```python
from build123d import *

# Parameters (mm, degrees)
F0_R           = 63.5
F1_DEPTH       = 12.7
F3_DEPTH       = 25.4
F4_D           = 6.35
F4_CBORE_D     = 10.3124
F4_CBORE_DEPTH = 6.35


# Not quite as in the source:
# - a feature names something its author has since deleted; it is built from what else it names


with BuildPart() as f1:
    # F0 (on Front) → F1 (new body)
    with BuildSketch(Plane.XZ):
        Circle(F0_R)
    extrude(amount=F1_DEPTH)

    # F2 (on face) → F3 (cut)
    with BuildSketch(Plane.XZ.offset(12.7)):
        with BuildLine():
            Line((-10.3124, 62.6570379625), (-6.35, 50.8))
            Line((-6.35, 50.8), (-6.35, -25.4))
            ThreePointArc((-6.35, -25.4), (0, -31.75), (6.35, -25.4))
            Line((6.35, -25.4), (6.35, 50.8))
            Line((6.35, 50.8), (10.3124, 62.6570379625))
            ThreePointArc((10.3124, 62.6570379625), (0, 63.5), (-10.3124, 62.6570379625))
        make_face()
    extrude(amount=-F3_DEPTH, mode=Mode.SUBTRACT)

    # F4 (through all)
    with Locations(Plane(origin=(0, 0, 0), x_dir=(1, 0, 0), z_dir=(0, 1, 0))):
        with Locations((44.45, -29.36875), (-44.45, -29.36875), (44.45, 29.36875), (-44.45, 29.36875)):
            CounterBoreHole(F4_D / 2, F4_CBORE_D / 2, F4_CBORE_DEPTH)


solid = f1.part
```
Work out the finished part from the listing and answer in its coordinate system (mm). A direction names the side the tool comes from. Round coordinates to 2 decimals unless told otherwise and drop trailing zeros. Order: outer loops, then holes, each group sorted by start corner. A loop starts at its lowest first (then second) coordinate and runs counter-clockwise, first axis right, second up.
Q1. A cutting plane is placed at A-A, the plane z = 0. Determine the outline of the cut face in (x, y), then the cut area to 3 significant figures.
Solution:
outline: (-63.5, -12.7) - (-6.35, -12.7) - (-6.35, 0) - (-63.5, 0) - close; (6.35, -12.7) - (63.5, -12.7) - (63.5, 0) - (6.35, 0) - close
area: 1,450 mm2
Q2. A tool of negligible diameter and unlimited length cuts with its end or side. For faces 5 (the cylindrical face through (-39.69, -3.13, -27.39)), 6 (the cylindrical face through (-41.28, -9.57, 29.23)), 7 (the flat face through (8.303, -6.439, 56.646)), from which of +Z, -Z, +X, -X, +Y, -Y can it reach the whole face along a straight path? Write none if from no direction.
Solution:
face 5: +Y
face 6: +Y, -Y
face 7: +Z, +Y, -Y
Q3. Find the intervals of material crossed by line 1 along Z through (x, y) = (-44.45, -9.25); line 2 along Z through (x, y) = (-44.45, -2.5); line 3 along X through (y, z) = (-6, 28), in increasing order.
Solution:
line 1: z = -45.35 to -32.54, -26.19 to 26.19, 32.54 to 45.35
line 2: z = -45.35 to -34.52, -24.21 to 24.21, 34.52 to 45.35
line 3: x = -56.99 to -49.42, -39.48 to -6.35, 6.35 to 39.48, 49.42 to 56.99
Q4. The mould has two halves that part along Z. Classify faces 1 (the cylindrical face through (41.42, -9.57, -30.32)), 2 (the flat face through (13, 0, 0)), 3 (the cylindrical face through (-2.647, -6.261, -63.445)), 4 (the flat face through (-8.36, -6.44, 56.81)): pulls with the +Z half, pulls with the -Z half, needs draft (parallel to the pull), parting line crosses it, or undercut.
Solution:
face 1: undercut
face 2: needs draft
face 3: parting line crosses it
face 4: pulls with the +Z half
Q5. A cutting plane is placed at B-B, the plane x = 44.45. Determine the outline of the cut face in (y, z), then the cut area to 3 significant figures.
Solution:
outline: (-12.7, -45.35) - (0, -45.35) - (0, -34.52) - (-6.35, -34.52) - (-6.35, -32.54) - (-12.7, -32.54) - close; (-12.7, -26.19) - (-6.35, -26.19) - (-6.35, -24.21) - (0, -24.21) - (0, 24.21) - (-6.35, 24.21) - (-6.35, 26.19) - (-12.7, 26.19) - close; (-12.7, 32.54) - (-6.35, 32.54) - (-6.35, 34.52) - (0, 34.52) - (0, 45.35) - (-12.7, 45.35) - close
area: 940 mm2
Q6. A cutting plane is placed at D-D, the plane x = -46. Determine the outline of the cut face in (y, z) (3 decimals).
Solution:
outline: (-12.7, -43.775) - (0, -43.775) - (0, -34.286) - (-6.35, -34.286) - (-6.35, -32.14) - (-12.7, -32.14) - close; (-12.7, -26.598) - (-6.35, -26.598) - (-6.35, -24.451) - (0, -24.451) - (0, 24.451) - (-6.35, 24.451) - (-6.35, 26.598) - (-12.7, 26.598) - close; (-12.7, 32.14) - (-6.35, 32.14) - (-6.35, 34.286) - (0, 34.286) - (0, 43.775) - (-12.7, 43.775) - close
Q7. A cutting plane is placed at C-C, the plane y = -2.75. Determine the outline of the cut face in (x, z), then the cut area to 3 significant figures.
Solution:
outline: (-10.31, 62.66) arc R63.5 ccw (long way) to (10.31, 62.66) - (6.35, 50.8) - (6.35, -25.4) arc R6.35 cw to (-6.35, -25.4) - (-6.35, 50.8) - close; hole circle Ø10.31 at (-44.45, -29.37); hole circle Ø10.31 at (-44.45, 29.37); hole circle Ø10.31 at (44.45, -29.37); hole circle Ø10.31 at (44.45, 29.37)
area: 11,100 mm2
Q8. Given pin 1 Ø8 at (x, z) = (44.45, -29.37) entering from -Y; pin 2 Ø1.5 at (y, z) = (-2, -6.5) entering from +X; pin 3 Ø4 at (y, z) = (-6, 44) entering from -X; pin 4 Ø10 at (x, z) = (-44.45, -29.37) entering from +Y, each flat-ended and moving along its own axis, determine where each tip first touches the part or whether it passes through.
Solution:
pin 1: stops at y = -12.7
pin 2: stops at x = 63.24
pin 3: stops at x = -47.63
pin 4: stops at y = -6.35
